Verification items for the finished model (mm, model axes). Coordinates: 2 decimals unless noted, no trailing zeros. Order: outer loops, then holes, each group sorted by start corner. A loop starts at its lowest first (then second) coordinate and runs counter-clockwise, first axis right, second up. Notation, with made-up numbers: M 57,-5 L 66,-5 A26 ccw 66,19 Z; hole C 42.25,81.25 d5. An arc over 180 degrees is marked long. Return JSON: item names as keys, results as strings. Group by question number.
1. Gauge pin test, flat ends, axial feed: pin 1 (1.6 mm diameter, centred on x = 22, y = 5.5, fed in from +Z); pin 2 (1 mm diameter, centred on x = 18, y = 4.5, fed in from +Z); pin 3 (5 mm diameter, centred on y = 6.5, z = -5, fed in from +X). Record the tip position at first contact, or that the pin passes through.
2. Section check A-A, the plane y = 6.5. Record the cut outline in (x, z), plus the area to 3 significant figures.
3. Material ranges on line 1 along X through (y, z) = (3.5, 20), recorded low to high.
4. Section check B-B, the plane z = 25. Record the cut outline in (x, y), plus the area to 3 significant figures.
```python
from build123d import *

# Parameters (mm, degrees)
SKETCH1_W           = 34
SKETCH1_H           = 65.5
BOSS_EXTRUDE1_DEPTH = 9.5


with BuildPart() as part:
    # Sketch1 → Boss-Extrude1 (new body)
    with BuildSketch(Plane(origin=(0, 0, 0), x_dir=(1, 0, 0), z_dir=(0, 1, 0))):
        Rectangle(SKETCH1_W, SKETCH1_H)
        with BuildLine():
            Line((19, 32.75), (17, 32.75))
            Line((17, 32.75), (17, 30.75))
            Line((17, 30.75), (19, 30.75))
            ThreePointArc((19, 30.75), (20.414213562, 30.164213562), (21, 28.75))
            Line((21, 28.75), (23, 28.75))
            ThreePointArc((23, 28.75), (21.828427125, 31.578427125), (19, 32.75))
        make_face()
    extrude(amount=BOSS_EXTRUDE1_DEPTH)


solid = part.part
```
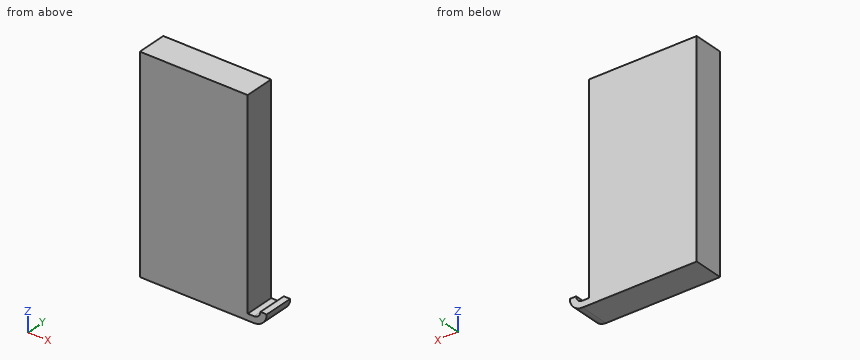
Answers follow:
{
 "1": {"pin 1": "z = -28.75", "pin 2": "z = -30.75", "pin 3": "x = 17"},
 "2": {"outline": "M -17,-32.75 L 19,-32.75 A4 ccw 23,-28.75 L 21,-28.75 A2 cw 19,-30.75 L 17,-30.75 L 17,32.75 L -17,32.75 Z", "area": "2,240 mm^2"},
 "3": {"line 1": "-17 to 17"},
 "4": {"outline": "M -17,0 L 17,0 L 17,9.5 L -17,9.5 Z", "area": "323 mm^2"}
}
